Autodesk Inventor part; units mm, degrees
ref_plane "Work Plane2" through (-89, -40.3889, 33.5) normal (0, 0, 1) x (1, 0, 0)
ref_plane "YZ Plane" through (0, 0, 0) normal (1, 0, 0) x (0, 1, 0)
ref_plane "XZ Plane" through (0, 0, 0) normal (0, 1, 0) x (-1, 0, 0)
ref_plane "Work Plane1" through (0, 0, 0) normal (0, 0, 1) x (1, 0, 0)
sketch "Sketch1" plane through (0, 0, 0) normal (0, 0, 1) x (1, 0, 0)
  line L0 (23.5, 88.5) -> (-23.5, 88.5)
  line L1 (-23.5, 88.5) -> (-23.5, 36.5)
  line L2 (-26.5, 33.5) -> (-89, 33.5)
  line L3 (-89, 33.5) -> (-89, -72.5)
  line L4 (-89, -72.5) -> (-77, -72.5)
  line L5 (-74, -75.5) -> (-74, -93.5)
  line L6 (-74, -93.5) -> (74, -93.5)
  line L7 (74, -93.5) -> (74, -75.5)
  line L8 (77, -72.5) -> (89, -72.5)
  line L9 (89, -72.5) -> (89, 33.5)
  line L10 (89, 33.5) -> (26.5, 33.5)
  line L11 (23.5, 36.5) -> (23.5, 88.5)
  line L12 (-4.5, 81.5) -> (-4.5, 36.5)
  line L13 (-7.5, 33.5) -> (-13.5, 33.5)
  line L14 (-16.5, 36.5) -> (-16.5, 81.5)
  line L15 (-13.5, 84.5) -> (-7.5, 84.5)
  line L16 (16.5, 81.5) -> (16.5, 36.5)
  line L17 (13.5, 33.5) -> (7.5, 33.5)
  line L18 (4.5, 36.5) -> (4.5, 81.5)
  line L19 (7.5, 84.5) -> (13.5, 84.5)
  line L20 (-16.5, 88.5) -> (-22.5, 88.5)
  line L21 (-22.5, 88.5) -> (-22.5, 3.75)
  line L22 (-22.5, 3.75) -> (-16.5, 3.75)
  line L23 (-16.5, 3.75) -> (-16.5, 88.5)
  line L24 (-32.2, 4.75) -> (-59.9, 4.75)
  arc A0 (13.5, 33.5) -> (16.5, 36.5) centre (13.5, 36.5) ccw
  arc A1 (4.5, 36.5) -> (7.5, 33.5) centre (7.5, 36.5) ccw
  arc A2 (7.5, 84.5) -> (4.5, 81.5) centre (7.5, 81.5) ccw
  arc A3 (16.5, 81.5) -> (13.5, 84.5) centre (13.5, 81.5) ccw
  arc A4 (-4.5, 81.5) -> (-7.5, 84.5) centre (-7.5, 81.5) ccw
  arc A5 (-7.5, 33.5) -> (-4.5, 36.5) centre (-7.5, 36.5) ccw
  arc A6 (-16.5, 36.5) -> (-13.5, 33.5) centre (-13.5, 36.5) ccw
  arc A7 (-13.5, 84.5) -> (-16.5, 81.5) centre (-13.5, 81.5) ccw
  arc A8 (-26.5, 33.5) -> (-23.5, 36.5) centre (-26.5, 36.5) ccw
  arc A9 (-74, -75.5) -> (-77, -72.5) centre (-77, -75.5) ccw
  arc A10 (77, -72.5) -> (74, -75.5) centre (77, -75.5) ccw
  arc A11 (23.5, 36.5) -> (26.5, 33.5) centre (26.5, 36.5) ccw
  point P0 (0, 0)
  point P1 (-16.5, 36.5)
  point P2 (-16.5, 81.5)
  dimension "d0" = 1
  dimension "d2" = 1
ref_plane "Work Plane2" through (-89, -40.3889, 33.5) normal (0, 0, 1) x (1, 0, 0)
extrude "Extrusion1" add sketch "Sketch1" along normal up to surface (33.5 mm away) contours L23 L14 L22 L21 L0
sketch "Sketch2" plane through (-22.5, 3.75, 0) normal (-1, 0, 0) x (0, 0, 1)
  arc A0 (13.7043, 8.7757) -> (14.863, 10.545) centre (10.3771, 12.2188) ccw
  arc A1 (14.863, 10.545) -> (15.4685, 10.512) centre (15.375, 14.375) ccw
  arc A2 (15.4685, 10.512) -> (16.4285, 8.6275) centre (20.1095, 11.6893) ccw
  arc A3 (16.4285, 8.6275) -> (17.3146, 8.863) centre (15.375, 14.375) ccw
  arc A4 (17.3146, 8.863) -> (17.2121, 10.9755) centre (12.599, 9.6929) ccw
  arc A5 (17.2121, 10.9755) -> (17.7212, 11.3047) centre (15.375, 14.375) ccw
  arc A6 (17.7212, 11.3047) -> (19.6056, 10.3444) centre (20.7839, 14.9851) ccw
  arc A7 (19.6056, 10.3444) -> (20.184, 11.0558) centre (15.375, 14.375) ccw
  arc A8 (20.184, 11.0558) -> (18.8594, 12.7045) centre (15.8813, 8.9554) ccw
  arc A9 (18.8594, 12.7045) -> (19.0778, 13.2702) centre (15.375, 14.375) ccw
  arc A10 (19.0778, 13.2702) -> (21.1668, 13.6008) centre (19.3923, 18.0479) ccw
  arc A11 (21.1668, 13.6008) -> (21.2166, 14.5164) centre (15.375, 14.375) ccw
  arc A12 (21.2166, 14.5164) -> (19.1758, 15.0716) centre (18.9701, 10.288) ccw
  arc A13 (19.1758, 15.0716) -> (19.02, 15.6576) centre (15.375, 14.375) ccw
  arc A14 (19.02, 15.6576) -> (20.5157, 17.153) centre (16.4662, 19.7077) ccw
  arc A15 (20.5157, 17.153) -> (20.0178, 17.923) centre (15.375, 14.375) ccw
  arc A16 (20.0178, 17.923) -> (18.0404, 17.1726) centre (20.6858, 13.1817) ccw
  arc A17 (18.0404, 17.1726) -> (17.57, 17.5552) centre (15.375, 14.375) ccw
  arc A18 (17.57, 17.5552) -> (17.9011, 19.644) centre (13.1233, 19.3306) ccw
  arc A19 (17.9011, 19.644) -> (17.0457, 19.9743) centre (15.375, 14.375) ccw
  arc A20 (17.0457, 19.9743) -> (15.887, 18.205) centre (20.3729, 16.5312) ccw
  arc A21 (15.887, 18.205) -> (15.2815, 18.238) centre (15.375, 14.375) ccw
  arc A22 (15.2815, 18.238) -> (14.3215, 20.1225) centre (10.6405, 17.0607) ccw
  arc A23 (14.3215, 20.1225) -> (13.4354, 19.887) centre (15.375, 14.375) ccw
  arc A24 (13.4354, 19.887) -> (13.5379, 17.7745) centre (18.151, 19.0571) ccw
  arc A25 (13.5379, 17.7745) -> (13.0288, 17.4453) centre (15.375, 14.375) ccw
  arc A26 (13.0288, 17.4453) -> (11.1444, 18.4056) centre (9.9661, 13.7649) ccw
  arc A27 (11.1444, 18.4056) -> (10.566, 17.6942) centre (15.375, 14.375) ccw
  arc A28 (10.566, 17.6942) -> (11.8906, 16.0455) centre (14.8687, 19.7946) ccw
  arc A29 (11.8906, 16.0455) -> (11.6722, 15.4798) centre (15.375, 14.375) ccw
  arc A30 (11.6722, 15.4798) -> (9.5832, 15.1492) centre (11.3577, 10.7021) ccw
  arc A31 (9.5832, 15.1492) -> (9.5334, 14.2336) centre (15.375, 14.375) ccw
  arc A32 (9.5334, 14.2336) -> (11.5742, 13.6784) centre (11.7799, 18.462) ccw
  arc A33 (11.5742, 13.6784) -> (11.73, 13.0924) centre (15.375, 14.375) ccw
  arc A34 (11.73, 13.0924) -> (10.2343, 11.597) centre (14.2838, 9.0423) ccw
  arc A35 (10.2343, 11.597) -> (10.7322, 10.827) centre (15.375, 14.375) ccw
  arc A36 (10.7322, 10.827) -> (12.7096, 11.5774) centre (10.0642, 15.5683) ccw
  arc A37 (12.7096, 11.5774) -> (13.18, 11.1948) centre (15.375, 14.375) ccw
  arc A38 (13.18, 11.1948) -> (12.8489, 9.106) centre (17.6267, 9.4194) ccw
  arc A39 (12.8489, 9.106) -> (13.7043, 8.7757) centre (15.375, 14.375) ccw
  circle A40 centre (15.375, 14.375) radius 6.75
  circle A41 centre (15.375, 14.375) radius 5.8433
  line L0 (21.2183, 14.375) -> (22.125, 14.375)
  circle A42 centre (10.5, 57.25) radius 5.5
  point P0 (0, -3.75)
  dimension "d6" = 13.5
  dimension "d5" = 0.9067
  dimension "d9" = 11
extrude "Extrusion2" cut sketch "Sketch2" against normal up to next contours A39 A38 A37 A36 A35 A34 A33 A32 A31 A30 A29 A28 A27 A26 A25 A24 A23 A22 A21 A20 A19 A18 A17 A16 A15 A14 A13 A12 A11 A10 A9 A8 A7 A6 A5 A4 A3 A2 A1 A0 | A0 A1 A2 A41 | A41 A36 A37 A38 | A4 A5 A6 A41 | A41 A32 A33 A34 | A8 A9 A10 A41 | A41 A28 A29 A30 | A41 A24 A25 A26 | A12 A13 A14 A41 | A41 A20 A21 A22 | A16 A17 A18 A41 | A40 | A42
sketch "Sketch3" plane through (-16.5, 3.75, 0) normal (1, 0, 0) x (0, 0, -1)
  circle A0 centre (-21.2694, 29.2497) radius 2
  point P0 (0, -3.75)
extrude "Extrusion3" cut sketch "Sketch3" against normal blind 5
ref_plane "Work Plane3" through (-23.5, 3.75, 0) normal (-1, 0, 0) x (0, 0, 1)
sketch "Sketch5" plane through (-23.5, 3.75, 0) normal (-1, 0, 0) x (0, 0, 1)
  circle A0 centre (29.5, 80.75) radius 2.1
  circle A1 centre (4, 80.75) radius 2.1
  circle A2 centre (3.5, 33.25) radius 2.1
  point P0 (0, -3.75)
hole "Hole1" at (-23.5, 84.5, 29.5) at (-23.5, 84.5, 4) at (-23.5, 37, 3.5) direction (1, 0, 0) diameter 3.6 end through all countersink diameter 6.2 countersink angle 90
sketch "Sketch6" plane through (-22.5, 3.75, 33.5) normal (0, 0, 1) x (1, 0, 0)
  line L0 (0, 7.625) -> (0, 21.125)
  line L1 (1, 31.2497) -> (1, 27.2497)
  line L2 (0, 31.15) -> (0, 35.35)
  line L3 (0, 51.75) -> (0, 62.75)
  line L4 (0, 78.65) -> (0, 82.85)
  line L5 (0, 78.65) -> (0, 82.85)
  line L6 (6, 0) -> (0, 0)
  line L7 (6, 84.75) -> (6, 0)
  line L8 (0, 84.75) -> (6, 84.75)
  line L9 (0, 0) -> (0, 84.75)
  line L10 (6, 27.125) -> (0, 27.125)
  line L11 (0, 27.125) -> (0, 35.35)
  line L12 (0, 35.35) -> (6, 35.35)
  line L13 (6, 35.35) -> (6, 27.125)
  line L14 (0, 7.625) -> (6, 7.625)
  line L15 (6, 7.625) -> (0, 7.625)
  line L16 (0, 7.625) -> (0, 21.125)
  line L17 (0, 21.125) -> (6, 21.125)
  line L18 (6, 21.125) -> (6, 7.625)
  line L19 (6, 78.95) -> (0.3, 78.95)
  line L20 (6, 84.75) -> (0, 84.75)
  line L21 (6, 78.95) -> (0, 78.95)
  line L22 (0, 78.95) -> (0, 84.75)
  line L23 (0, 84.75) -> (6, 84.75)
  line L24 (6, 84.75) -> (6, 78.95)
  line L25 (0, 51.75) -> (6, 51.75)
  line L26 (0, 51.75) -> (0, 62.75)
  line L27 (6, 51.75) -> (0, 51.75)
  line L28 (0, 51.75) -> (0, 62.75)
  line L29 (0, 62.75) -> (6, 62.75)
  line L30 (6, 62.75) -> (6, 51.75)
  line L31 (6, 0) -> (0, 0)
  line L32 (0, 0) -> (0, 3.7)
  line L33 (0, 3.7) -> (6, 3.7)
  line L34 (6, 3.7) -> (6, 0)
  circle A0 centre (3, 5.5) radius 1.8
  line L35 (6, 21.125) -> (0, 27.125)
  line L36 (0, 21.125) -> (6, 27.125)
  line L37 (6, 35.35) -> (0, 51.75)
  line L38 (0, 35.35) -> (6, 51.75)
  line L39 (0.3, 82.55) -> (0.3, 78.95)
  line L40 (6, 62.75) -> (0.3, 78.95)
  line L41 (6, 82.55) -> (6, 78.95)
  line L42 (0.3, 78.95) -> (6, 78.95)
  line L43 (6, 78.95) -> (0, 62.75)
  point P0 (22.5, -3.75)
  point P1 (3, 24.125)
  point P2 (3.0769, 71.0577)
  point P3 (3, 43.55)
  dimension "d20" = 3.7
  dimension "d21" = 3.6
  dimension "d22" = 3
  dimension "d23" = 3
hole "Hole2" at (-19.5, 27.875, 33.5) at (-19.5, 9.25, 33.5) at (-19.4231, 74.8077, 33.5) at (-19.5, 47.3, 33.5) direction (0, 0, -1) diameter 3.6 end through all countersink diameter 6.3 countersink angle 90
sketch "Sketch7" plane through (-22.5, 3.75, 0) normal (0, -1, 0) x (1, 0, 0)
  line L0 (6, 33.5) -> (0, 33.5)
  line L1 (0, 0) -> (0, 33.5)
  line L2 (0, 0) -> (6, 0)
  line L3 (6, 0) -> (6, 33.5)
  line L4 (0, 0) -> (0, 33.5)
  line L5 (0, 16.75) -> (6, 16.75)
  line L6 (6, 16.75) -> (0, 33.5)
  line L7 (6, 16.75) -> (0, 0)
  line L8 (6, 0) -> (0, 0)
  line L9 (6, 0) -> (0, 16.75)
  line L10 (0, 33.5) -> (6, 33.5)
  line L11 (6, 33.5) -> (0, 16.75)
  point P0 (22.5, 0)
  point P1 (3, 25.125)
  point P2 (3, 8.375)
hole "Hole3" at (-19.5, 3.75, 25.125) at (-19.5, 3.75, 8.375) direction (0, 1, 0) diameter 4 depth 3.6 counterbore diameter 4.6 counterbore depth 0.6
sketch "Sketch9" plane through (-22.5, 88.5, 0) normal (0, 1, 0) x (1, 0, 0)
  circle A0 centre (22.5, -20.825) radius 2.3
  circle A1 centre (22.5, -12.675) radius 2.3
  line L0 (18, -33.5) -> (27, -33.5)
  line L1 (27, 0) -> (27, -33.5)
  line L2 (27, 0) -> (18, 0)
  line L3 (18, 0) -> (18, -33.5)
  line L4 (22.5, -20.825) -> (0, -20.825)
  line L5 (0, -22.125) -> (0, -8.625)
  line L6 (22.5, -12.675) -> (0, -12.675)
  line L7 (6, 0) -> (6, -33.5)
  point P0 (22.5, 0)
  point P1 (3, -20.825)
  point P2 (3, -12.675)
  dimension "d45" = 3
  dimension "d46" = 3
  dimension "d47" = 3
  dimension "d48" = 3
hole "Hole5" at (-19.5, 88.5, 20.825) at (-19.5, 88.5, 12.675) direction (0, -1, 0) diameter 4 depth 6 counterbore diameter 4.6 counterbore depth 1.5
sketch "Sketch10" plane through (-19.5, 47.3, 33.5) normal (0, 0, 1) x (1, 0, 0)
  line L0 (-3, 8.2) -> (-3, 19.2)
  arc A0 (3, -18.4645) -> (-3, -18.4645) centre (0, -19.425) ccw
  arc A1 (-3, -0.9605) -> (3, -0.9605) centre (0, 0) ccw
  arc A2 (3, -18.4645) -> (-3, -18.4645) centre (0, -19.425) ccw
  line L1 (3, -0.9605) -> (3, -18.4645)
  arc A3 (-3, -0.9605) -> (3, -0.9605) centre (0, 0) ccw
  line L2 (-3, -18.4645) -> (-3, -0.9605)
  line L3 (3, 8.2) -> (-3, 8.2)
  line L4 (3, 19.2) -> (-3, 19.2)
  line L5 (-3, 19.2) -> (3, 8.2)
  line L6 (-3, 8.2) -> (3, 19.2)
  line L7 (3, -18.4645) -> (-3, -0.9605)
  line L8 (-3, -18.4645) -> (3, -0.9605)
  point P0 (19.5, -47.3)
  point P1 (0, -9.7125)
  point P2 (0, 13.7)
hole "Hole6" at (-19.5, 37.5875, 33.5) at (-19.5, 61, 33.5) direction (0, 0, -1) diameter 4 depth 6 counterbore diameter 4.6 counterbore depth 1.5
equation "\"d22\" = d23"
properties part number "right_gear_holder"
Build history of the part. All positions in model axes, mm. A direction names the side the tool comes from. Coordinates: 2 decimals unless noted, no trailing zeros. Order: outer loops, then holes, each group sorted by start corner. A loop starts at its lowest first (then second) coordinate and runs counter-clockwise, first axis right, second up.
Item 1: Saw through at A-A on y = 61. List the corners of the cut face in (x, z).
Filled in:
outline: (-22.5, 0) - (-16.5, 0) - (-16.5, 5) - (-22.5, 5) - close; (-22.5, 16) - (-16.5, 16) - (-16.5, 33.5) - (-17.2, 33.5) - (-17.2, 32) - (-17.5, 32) - (-17.5, 27.5) - (-21.5, 27.5) - (-21.5, 32) - (-21.8, 32) - (-21.8, 33.5) - (-22.5, 33.5) - close
Item 2: Drop flat-ended pins along their axis: pin 1 Ø3 at (x, z) = (-19, 13.5) entering from +Y; pin 2 Ø2.5 at (x, z) = (-20, 21) entering from +Y; pin 3 Ø2.5 at (x, z) = (-18.5, 25) entering from -Y; pin 4 Ø1.4 at (x, y) = (-20.5, 60) entering from +Z. Give the stop position or say it passes through.
Filled in:
pin 1: stops at y = 88.5
pin 2: stops at y = 82.5
pin 3: stops at y = 4.35
pin 4: stops at z = 32
Item 3: Saw through at B-B on z = 12. State how many separate pieces and enclosed holes the cut face has, then the cut area to 3 significant figures.
Filled in:
separate pieces: 3
enclosed holes: 4
area: 311 mm2
Item 4: Tool access for faces 5 (the flat face through (-21.5, 33, 21)), 6 (the flat face through (-16.5, 46, 17)), 7 (the cylindrical face through (-17.46, 59.94, 32.74)), 8 (the cylindrical face through (-21.483, 5.871, 8.635)), 9 (the cylindrical face through (-21, 85, 14)): list every direction of +Z, -Z, +X, -X, +Y, -Y with a clear straight run to the whole face (end or side of a thin tool).
Filled in:
face 5: +X
face 6: +Z, -Z, +X, +Y, -Y
face 7: +Z
face 8: -Y
face 9: +Y
Item 5: Mould opens along Z. For faces 1 (the flat face through (-22, 47, 0)), 2 (the flat face through (-20, 3.75, 17)), 3 (the flat face through (-20, 82.5, 13)), 4 (the flat face through (-20, 5, 33.5)) say: released by +Z, released by -Z, zero draft, split by the parting line, or undercut.
Filled in:
face 1: released by -Z
face 2: zero draft
face 3: undercut
face 4: released by +Z
Item 6: Drill centre lines: L1, parallel to Z at x = -19.5, y = 87.75 (3 decimals); L2, parallel to Z at x = -19.5, y = 84.7 (3 decimals); L3, parallel to Z at x = -19.5, y = 4.1 (3 decimals). Where is each one in solid material? Low to high.
Filled in:
L1: z = 0 to 10.375, 14.975 to 18.525, 23.125 to 33.5
L2: z = 0 to 2.211, 5.789 to 10.675, 14.675 to 18.825, 22.825 to 27.711, 31.289 to 33.5
L3: z = 0 to 6.075, 10.675 to 22.825, 27.425 to 33.5
